from build123d import *

# Parameters (mm, degrees)
SKETCH_1_W                        = 1500
SKETCH_1_H                        = 262
EXTRUDE_1_DEPTH                   = 200
SKETCH_5_W                        = 232
SKETCH_5_H                        = 238
SKETCH_5_W_2                      = 488
CUT_EXTRUDE_10_DEPTH              = 1536.787745751
SKETCH_7_W                        = 1500
SKETCH_7_H                        = 12
EXTRUDE_13_DEPTH                  = 260
SKETCH_8_R                        = 11
CUT_EXTRUDE_14_DEPTH              = 1536.787745751
PATTERN_LINEAR_3_COUNT            = 12
PATTERN_LINEAR_3_PITCH            = 125
PATTERN_LINEAR_3_COUNT_DIR2       = 2
PATTERN_LINEAR_3_PITCH_DIR2       = 125
SKETCH_10_R                       = 11
CUT_EXTRUDE_16_DEPTH              = 20
PATTERN_LINEAR_5_COUNT            = 2
PATTERN_LINEAR_5_PITCH            = 125
PATTERN_LINEAR_5_COUNT_DIR2       = 2
PATTERN_LINEAR_5_PITCH_DIR2       = 125
CUT_EXTRUDE_START                 = -20
SKETCH_11_R                       = 11
CUT_EXTRUDE_17_DEPTH              = 20
PATTERN_LINEAR_6_COUNT            = 2
PATTERN_LINEAR_6_PITCH            = 125
PATTERN_LINEAR_6_COUNT_DIR2       = 2
PATTERN_LINEAR_6_PITCH_DIR2       = 125
SKETCH_12_R                       = 11
CUT_EXTRUDE_18_DEPTH              = 1050
PATTERN_LINEAR_8_COUNT            = 2
PATTERN_LINEAR_8_PITCH            = 140.2426687
FILLET_1_R                        = 10
FILLET_2_R                        = 10
SKETCH_13_R                       = 11
CUT_EXTRUDE_19_DEPTH              = 1527.394444434
PATTERN_LINEAR_9_COUNT            = 2
PATTERN_LINEAR_9_PITCH            = 125
PATTERN_LINEAR_9_COUNT_DIR2       = 2
PATTERN_LINEAR_9_PITCH_DIR2       = 125
PATTERN_LINEAR_10_COUNT           = 2
PATTERN_LINEAR_10_PITCH           = 500
PATTERN_LINEAR_10_COPY_1_SKETCH_R = 11
PATTERN_LINEAR_10_COPY_1_DEPTH    = 1527.394444434
PATTERN_LINEAR_10_COPY_2_SKETCH_R = 11
PATTERN_LINEAR_10_COPY_2_DEPTH    = 1527.394444434
PATTERN_LINEAR_10_COPY_3_SKETCH_R = 11
PATTERN_LINEAR_10_COPY_3_DEPTH    = 1527.394444434


with BuildPart() as part:
    # 草图1 → 拉伸1 (new body)
    with BuildSketch(Plane.XY):
        with Locations((750, 131)):
            Rectangle(SKETCH_1_W, SKETCH_1_H)
    extrude(amount=EXTRUDE_1_DEPTH)

    # 草图5 → 拉伸10 (cut, through all)
    with BuildSketch(Plane.XY.offset(200)):
        with Locations((128, 131)):
            Rectangle(SKETCH_5_W, SKETCH_5_H)
        with Locations((500, 131)):
            Rectangle(SKETCH_5_W_2, SKETCH_5_H)
        with Locations((1000, 131)):
            Rectangle(SKETCH_5_W_2, SKETCH_5_H)
        with Locations((1372, 131)):
            Rectangle(SKETCH_5_W, SKETCH_5_H)
    extrude(amount=-CUT_EXTRUDE_10_DEPTH, mode=Mode.SUBTRACT)

    # 草图7 → 拉伸13 (add)
    with BuildSketch(Plane.XZ):
        with Locations((750, 100)):
            Rectangle(SKETCH_7_W, SKETCH_7_H)
    extrude(amount=-EXTRUDE_13_DEPTH)

    # 草图8 → 拉伸14 (cut, through all)
    with BuildSketch(Plane.XZ):
        with Locations(Location((62.5, 37.5, 0), (0, 0, 270))):
            Circle(SKETCH_8_R)
    cut_extrude_14 = extrude(amount=-CUT_EXTRUDE_14_DEPTH, mode=Mode.SUBTRACT)

    # 阵列(线性)3: Cut-Extrude 14 12 × 2
    with Locations(*[(i * PATTERN_LINEAR_3_PITCH, 0, j * PATTERN_LINEAR_3_PITCH_DIR2) for i in range(PATTERN_LINEAR_3_COUNT) for j in range(PATTERN_LINEAR_3_COUNT_DIR2) if (i, j) != (0, 0)]):
        add(cut_extrude_14, mode=Mode.SUBTRACT)

    # 草图10 → 拉伸16 (cut)
    with BuildSketch(Plane.ZY):
        with Locations((37.5, 68.5)):
            Circle(SKETCH_10_R)
    cut_extrude_16 = extrude(amount=-CUT_EXTRUDE_16_DEPTH, mode=Mode.SUBTRACT)

    # 阵列(线性)5: Cut-Extrude 16 2 × 2
    with Locations(*[(0, j * PATTERN_LINEAR_5_PITCH_DIR2, i * PATTERN_LINEAR_5_PITCH) for i in range(PATTERN_LINEAR_5_COUNT) for j in range(PATTERN_LINEAR_5_COUNT_DIR2) if (i, j) != (0, 0)]):
        add(cut_extrude_16, mode=Mode.SUBTRACT)

    # 草图11 → 拉伸17 (cut)
    with BuildSketch(Plane(origin=(1500, 0, 0), x_dir=(0, 0, -1), z_dir=(1, 0, 0)).offset(CUT_EXTRUDE_START)):
        with Locations(Location((-162.5, 68.5, 0), (0, 0, 180))):
            Circle(SKETCH_11_R)
    cut_extrude_17 = extrude(amount=CUT_EXTRUDE_17_DEPTH, mode=Mode.SUBTRACT)

    # 阵列(线性)6: Cut-Extrude 17 2 × 2
    with Locations(*[(0, j * PATTERN_LINEAR_6_PITCH_DIR2, -i * PATTERN_LINEAR_6_PITCH) for i in range(PATTERN_LINEAR_6_COUNT) for j in range(PATTERN_LINEAR_6_COUNT_DIR2) if (i, j) != (0, 0)]):
        add(cut_extrude_17, mode=Mode.SUBTRACT)

    # 草图12 → 拉伸18 (cut)
    with BuildSketch(Plane(origin=(1256, 0, 0), x_dir=(0, 0, -1), z_dir=(1, 0, 0))):
        with Locations((-170.12133435, 131)):
            Circle(SKETCH_12_R)
    cut_extrude_18 = extrude(amount=-CUT_EXTRUDE_18_DEPTH, mode=Mode.SUBTRACT)

    # 阵列(线性)8: 拉伸18 ×2
    with Locations(*[(0, 0, -i * PATTERN_LINEAR_8_PITCH) for i in range(1, PATTERN_LINEAR_8_COUNT)]):
        add(cut_extrude_18, mode=Mode.SUBTRACT)

    # 圆角1
    fillet_1_edges = [part.edges().sort_by_distance(p)[0] for p in [
        (0, 131, 200),
        (0, 131, 0),
        (0, 262, 100),
        (0, 0, 100),
    ]]
    fillet(fillet_1_edges, radius=FILLET_1_R)

    # 圆角2
    fillet_2_edges = [part.edges().sort_by_distance(p)[0] for p in [
        (1500, 131, 200),
        (1500, 131, 0),
        (1500, 262, 100),
        (1500, 0, 100),
    ]]
    fillet(fillet_2_edges, radius=FILLET_2_R)

    # 草图13 → 拉伸19 (cut, through all)
    with BuildSketch(Plane.XY.offset(106)):
        with Locations((437.5, 68.5)):
            Circle(SKETCH_13_R)
    cut_extrude_19 = extrude(amount=-CUT_EXTRUDE_19_DEPTH, mode=Mode.SUBTRACT)

    # 阵列(线性)9: Cut-Extrude 19 2 × 2
    with Locations(*[(i * PATTERN_LINEAR_9_PITCH, j * PATTERN_LINEAR_9_PITCH_DIR2, 0) for i in range(PATTERN_LINEAR_9_COUNT) for j in range(PATTERN_LINEAR_9_COUNT_DIR2) if (i, j) != (0, 0)]):
        add(cut_extrude_19, mode=Mode.SUBTRACT)

    # 阵列(线性)10: 拉伸19 ×2
    with Locations(*[(i * PATTERN_LINEAR_10_PITCH, 0, 0) for i in range(1, PATTERN_LINEAR_10_COUNT)]):
        add(cut_extrude_19, mode=Mode.SUBTRACT)

    # 阵列(线性)10 copy 1 sketch → 阵列(线性)10 copy 1 (cut, through all)
    with BuildSketch(Plane(origin=(500, 125, 106), x_dir=(1, 0, 0), z_dir=(0, 0, 1))):
        with Locations((437.5, 68.5)):
            Circle(PATTERN_LINEAR_10_COPY_1_SKETCH_R)
    extrude(amount=-PATTERN_LINEAR_10_COPY_1_DEPTH, mode=Mode.SUBTRACT)

    # 阵列(线性)10 copy 2 sketch → 阵列(线性)10 copy 2 (cut, through all)
    with BuildSketch(Plane(origin=(625, 0, 106), x_dir=(1, 0, 0), z_dir=(0, 0, 1))):
        with Locations((437.5, 68.5)):
            Circle(PATTERN_LINEAR_10_COPY_2_SKETCH_R)
    extrude(amount=-PATTERN_LINEAR_10_COPY_2_DEPTH, mode=Mode.SUBTRACT)

    # 阵列(线性)10 copy 3 sketch → 阵列(线性)10 copy 3 (cut, through all)
    with BuildSketch(Plane(origin=(625, 125, 106), x_dir=(1, 0, 0), z_dir=(0, 0, 1))):
        with Locations((437.5, 68.5)):
            Circle(PATTERN_LINEAR_10_COPY_3_SKETCH_R)
    extrude(amount=-PATTERN_LINEAR_10_COPY_3_DEPTH, mode=Mode.SUBTRACT)


solid = part.part
The model under review builds one solid part; all positions refer to its coordinate system, in mm. A direction names the side the tool comes from. Round coordinates to 2 decimals unless told otherwise and drop trailing zeros. Loops run counter-clockwise (first coordinate to the right, second up) from the corner with the lowest first, then second, coordinate; pieces in that order, holes last. Notation, with made-up numbers: M -23,36.25 L 23,36.25 A13 ccw 23,61.25 Z; hole C 38,1 d6. An arc over 180 degrees is marked long. Answer as a JSON object with one key per item and string values.
Item 1: We need section A-A, the plane z = 81. State the section outline as (x, y) points, and give its area (3 significant figures).
Check sheet entries:
{"outline": "M 0,10 A10 ccw 10,0 L 1490,0 A10 ccw 1500,10 L 1500,252 A10 ccw 1490,262 L 10,262 A10 ccw 0,252 Z; hole M 12,12 L 244,12 L 244,250 L 12,250 Z; hole M 256,12 L 744,12 L 744,250 L 256,250 Z; hole M 756,12 L 1244,12 L 1244,250 L 756,250 Z; hole M 1256,12 L 1488,12 L 1488,250 L 1256,250 Z", "area": "50,200 mm2"}
Item 2: We need section B-B, the plane x = 861.5. State the section outline as (y, z) points.
Check sheet entries:
{"outline": "M 0,0 L 12,0 L 12,94 L 250,94 L 250,0 L 262,0 L 262,200 L 250,200 L 250,106 L 12,106 L 12,200 L 0,200 Z"}
Item 3: Clearance check with a flat-ended pin moving along its axis: P1, Ø1.5, axis at x = 373, y = 186, coming from the -Z side. State where the tip first meets the part, or that it passes through.
Check sheet entries:
{"P1": "z = 94"}
Item 4: For line 1 along Z through (x, y) = (562.5, 5); line 2 along X through (y, z) = (208.5, 14); line 3 along X through (y, z) = (74, 31.5), list the stretches that pass through material, from the lowest coordinate up.
Check sheet entries:
{"line 1": "0 to 26.5, 48.5 to 151.5, 173.5 to 200", "line 2": "0 to 12, 244 to 256, 744 to 756, 1244 to 1256, 1488 to 1500", "line 3": "244 to 256, 744 to 756, 1244 to 1256"}
Item 5: Tool access review of faces 1 (the face through (1256, 129, 154)), 2 (the face through (997, 12, 48)): name each direction out of +Z, -Z, +X, -X, +Y, -Y from which nothing blocks a thin tool from reaching the whole face with its end or side.
Check sheet entries:
{"face 1": "+Z", "face 2": "-Z"}
Item 6: The part is to be moulded in two halves that separate along Y. For faces 3 (the face through (256, 129, 48)), 4 (the face through (747, 132, 200)), 5 (the face through (1488, 129, 48)), 6 (the face through (740, 0, 101)), say which applies: +Y half, -Y half, draft (parallel to the pull), parting line (faces both ways), or undercut.
Check sheet entries:
{"face 3": "undercut", "face 4": "draft", "face 5": "undercut", "face 6": "-Y half"}
